The figure shows three views and two pictorial views of one solid part (mm, origin at its lowest corner). Answer the questions. Coordinates: 2 decimals unless noted, no trailing zeros. Loops run counter-clockwise (first coordinate to the right, second up) from the corner with the lowest first, then second, coordinate; pieces in that order, holes last. Notation, with made-up numbers: (28, 26.5) - (52, 26.5) arc R17 ccw to (52, 53.5) - close; hole circle Ø6 at (-3.5, -14). An arc over 180 degrees is marked (long way). Return JSON: item names as keys, results as strings. Group by question number.
1. Section C-C (z = 0.1) is taken. Write down the section's boundary in (x, y).
2. Section B-B (x = 3) is taken. Write down the section's boundary in (y, z), and give its area (3 significant figures).
3. Find the intervals of material crossed by line 1 along X through (y, z) = (3, 0.15); line 2 along Y through (x, z) = (4.1, 0.15), in increasing order.
4. This flat-tipped pin is pushed along its axis until it touches: P1, Ø2, axis at x = 4, y = 1.5, coming from the -Z side. Where does it stop, or does it pass through?
5. Section A-A (y = 1.6) is taken. Write down the section's boundary in (x, z).
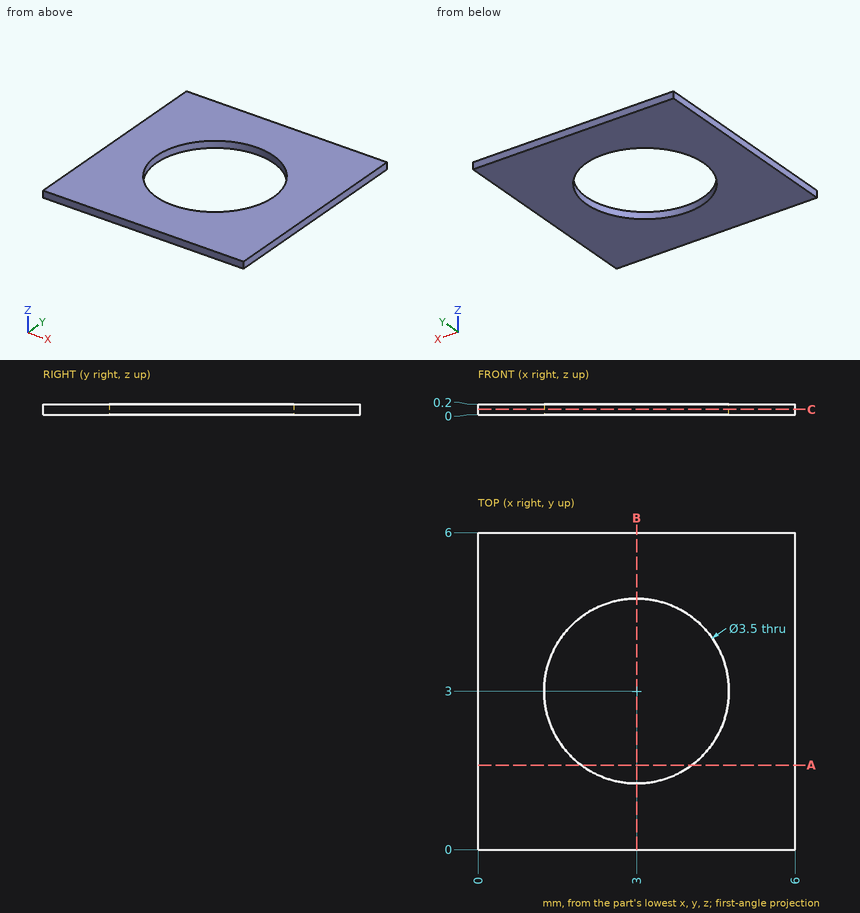
The answers:
{
 "1": {"outline": "(0, 0) - (6, 0) - (6, 6) - (0, 6) - close; hole circle Ø3.5 at (3, 3)"},
 "2": {"outline": "(0, 0) - (1.25, 0) - (1.25, 0.2) - (0, 0.2) - close; (4.75, 0) - (6, 0) - (6, 0.2) - (4.75, 0.2) - close", "area": "0.500 mm2"},
 "3": {"line 1": "x = 0 to 1.25, 4.75 to 6", "line 2": "y = 0 to 1.64, 4.36 to 6"},
 "4": {"P1": "stops at z = 0"},
 "5": {"outline": "(0, 0) - (1.95, 0) - (1.95, 0.2) - (0, 0.2) - close; (4.05, 0) - (6, 0) - (6, 0.2) - (4.05, 0.2) - close"}
}
